Build history of the part. All positions in model axes, mm. A direction names the side the tool comes from. Round coordinates to 2 decimals unless told otherwise and drop trailing zeros. Order: outer loops, then holes, each group sorted by start corner. A loop starts at its lowest first (then second) coordinate and runs counter-clockwise, first axis right, second up. Notation, with made-up numbers: (35, -11.5) -> (67, -11.5) arc R17 cw to (67, 3.5) -> close; hole circle Ø10 at (2, 88.5). An arc over 180 degrees is marked (long way). Answer as a JSON object with one key per item and string values.
from build123d import *

# Parameters (mm, degrees)
EXTRUDE_1_DEPTH         = 3
SKETCH_2_R              = 1.35
CUT_EXTRUDE_1_DEPTH     = 2.444444444
SKETCH_3_R              = 1.35
CUT_EXTRUDE_2_DEPTH     = 0.555555556
HOLE_WIZARD_2_7_2_7_1_D = 2.7
SKETCH_6_R              = 1.65
CUT_EXTRUDE_3_DEPTH     = 64.035907885
CUT_EXTRUDE_4_DEPTH     = 1


with BuildPart() as part:
    # 草图1 → 凸台-拉伸1 (new body)
    with BuildSketch(Plane.XY.offset(3)):
        with BuildLine():
            Line((23.778016459, 8.467622986), (-52.596358319, 8.467622986))
            ThreePointArc((-52.596358319, 8.467622986), (-62.214907854, 3.590303351), (-52.451603626, -0.990377005))
            Line((-52.451603626, -0.990377005), (23.856567017, 0.468594516))
            ThreePointArc((23.856567017, 0.468594516), (27.777721585, 4.50700022), (23.778016459, 8.467622986))
        make_face()
    extrude(amount=-EXTRUDE_1_DEPTH)

    # 草图2 → 切除-拉伸1 (cut)
    with BuildSketch(Plane.XY.offset(3)):
        with Locations(Location((23.77801746, 4.467622995, 0), (0, 0, 180))):
            Circle(SKETCH_2_R)
    extrude(amount=-CUT_EXTRUDE_1_DEPTH, mode=Mode.SUBTRACT)

    # 草图3 → 切除-拉伸2 (cut)
    with BuildSketch(Plane(origin=(0, 0, 0), x_dir=(-1, 0, 0), z_dir=(0, 0, -1))):
        with Locations(Location((-23.778017455, 4.467823177, 0), (0, 0, 359.991504025))):
            Circle(SKETCH_3_R)
    extrude(amount=-CUT_EXTRUDE_2_DEPTH, mode=Mode.SUBTRACT)

    # Ø2.7 (2.7) 直径孔1 (through all)
    with Locations(Plane.XY.offset(3)):
        with Locations((-56.215609969, 3.682122995)):
            Hole(HOLE_WIZARD_2_7_2_7_1_D / 2)

    # 草图6 → 切除-拉伸3 (cut, through all)
    with BuildSketch(Plane.XY.offset(3)):
        with Locations((-56.215609969, 3.682122995)):
            Circle(SKETCH_6_R)
        with Locations((23.778017455, 4.467823177)):
            Circle(SKETCH_6_R)
    extrude(amount=-CUT_EXTRUDE_3_DEPTH, mode=Mode.SUBTRACT)

    # 草图7 → 切除-拉伸4 (cut)
    with BuildSketch(Plane.XY.offset(3)):
        with BuildLine():
            Line((-28.902991884, 4.643891928), (-29.217094448, 4.643891928))
            add(Edge.make_bspline(
                [(-29.217094448, 4.643891928), (-29.208584898, 4.679124412), (-29.191949422, 4.748001036), (-29.157251849, 4.846408297), (-29.119452594, 4.939531818), (-29.074063489, 5.025627892), (-29.024554735, 5.106426795), (-28.967832013, 5.180095919), (-28.906512291, 5.248508885), (-28.838687341, 5.309222122), (-28.76755868, 5.364199852), (-28.69212406, 5.411074909), (-28.613901166, 5.451399062), (-28.532348033, 5.484619294), (-28.447221862, 5.509644817), (-28.359292238, 5.527801623), (-28.268328738, 5.539592737), (-28.206581148, 5.5407435), (-28.175227461, 5.541327825)],
                knots=[0, 0, 0, 0, 1.162005537, 2.271625781, 3.343758855, 4.383309926, 5.390229558, 6.379919256, 7.361854164, 8.333198761, 9.295911338, 10.242430842, 11.177959212, 12.116337295, 13.062827104, 14.020064771, 14.994644689, 16, 16, 16, 16], degree=3))
            add(Edge.make_bspline(
                [(-28.175227461, 5.541327825), (-28.129544719, 5.539948595), (-28.039175708, 5.53722022), (-27.906412661, 5.512305783), (-27.778385842, 5.472880651), (-27.656496594, 5.418406924), (-27.543278162, 5.35121961), (-27.442541975, 5.271254874), (-27.355653464, 5.180055572), (-27.282759087, 5.079323008), (-27.225684088, 4.971667498), (-27.183597714, 4.860867341), (-27.157976033, 4.74718537), (-27.154655476, 4.670428091), (-27.152991884, 4.631972857)],
                knots=[0, 0, 0, 0, 1.083050992, 2.142477498, 3.193116406, 4.255571735, 5.30263384, 6.308962982, 7.297363603, 8.282367274, 9.249857812, 10.179914175, 11.08814088, 12, 12, 12, 12], degree=3))
            add(Edge.make_bspline(
                [(-27.152991884, 4.631972857), (-27.154155475, 4.594966063), (-27.156432443, 4.522549508), (-27.175766148, 4.416828011), (-27.208302411, 4.317186411), (-27.253372174, 4.223205249), (-27.311713724, 4.135480409), (-27.382386421, 4.053814518), (-27.465889082, 3.97784536), (-27.52916802, 3.934325887), (-27.561745891, 3.911920774)],
                knots=[0, 0, 0, 0, 1.024540389, 2.004866551, 2.965041327, 3.920577974, 4.882998113, 5.874504559, 6.905732034, 8, 8, 8, 8], degree=3))
            add(Edge.make_bspline(
                [(-27.561745891, 3.911920774), (-27.524514136, 3.893942602), (-27.450747262, 3.858322645), (-27.350196732, 3.788466887), (-27.258918857, 3.70781054), (-27.208015138, 3.644867887), (-27.182439, 3.613242889)],
                knots=[0, 0, 0, 0, 1.015518401, 2.012035669, 3.001164323, 4, 4, 4, 4], degree=3))
            add(Edge.make_bspline(
                [(-27.182439, 3.613242889), (-27.165597657, 3.590185138), (-27.132190761, 3.544447221), (-27.090955228, 3.470910795), (-27.053546113, 3.396559306), (-27.024395894, 3.3193999), (-27.001822027, 3.240326886), (-26.985685995, 3.15920449), (-26.975661854, 3.075966468), (-26.974226302, 3.019653988), (-26.973504705, 2.991347857)],
                knots=[0, 0, 0, 0, 1.025084078, 2.033381695, 3.024893161, 4.013698104, 4.991890475, 5.976764909, 6.982997093, 8, 8, 8, 8], degree=3))
            add(Edge.make_bspline(
                [(-26.973504705, 2.991347857), (-26.975299218, 2.942338136), (-26.9788798, 2.844549334), (-27.010883875, 2.700074613), (-27.060497115, 2.55884911), (-27.130954051, 2.423774271), (-27.21682156, 2.29739389), (-27.318978884, 2.184317581), (-27.436265293, 2.087118977), (-27.567070942, 2.005908749), (-27.70878807, 1.940990827), (-27.860363662, 1.895933384), (-28.019613716, 1.866587384), (-28.128821014, 1.863440515), (-28.184342045, 1.861840646)],
                knots=[0, 0, 0, 0, 0.955779014, 1.907060117, 2.875433937, 3.871313158, 4.872415639, 5.851225146, 6.836215519, 7.83643374, 8.849228613, 9.86973379, 10.916971861, 12, 12, 12, 12], degree=3))
            add(Edge.make_bspline(
                [(-28.184342045, 1.861840646), (-28.221761345, 1.862708859), (-28.29539005, 1.864417213), (-28.403633548, 1.876095814), (-28.506955248, 1.89742582), (-28.605494846, 1.926129125), (-28.699339882, 1.962520867), (-28.788203987, 2.007839565), (-28.872633881, 2.061151067), (-28.951832832, 2.123084655), (-29.0257914, 2.192365995), (-29.092544124, 2.270225005), (-29.153203917, 2.355222409), (-29.206146555, 2.448345465), (-29.253783508, 2.548390722), (-29.292964465, 2.656639221), (-29.327450033, 2.772123243), (-29.343483498, 2.852600983), (-29.351709833, 2.893891928)],
                knots=[0, 0, 0, 0, 1.048658725, 2.063410685, 3.046034179, 4.001477787, 4.936774919, 5.862367409, 6.792675028, 7.730719943, 8.675894397, 9.627829632, 10.600096036, 11.597688215, 12.626045268, 13.701542398, 14.82072376, 16, 16, 16, 16], degree=3))
            Line((-29.351709833, 2.893891928), (-29.037607269, 2.893891928))
            add(Edge.make_bspline(
                [(-29.037607269, 2.893891928), (-29.029423978, 2.866942915), (-29.013506765, 2.814524743), (-28.986412467, 2.739084437), (-28.955544195, 2.669926384), (-28.922429636, 2.606543262), (-28.88765119, 2.54831086), (-28.848736265, 2.496768991), (-28.80856712, 2.449653788), (-28.778287766, 2.423109176), (-28.763468647, 2.410117889)],
                knots=[0, 0, 0, 0, 1.198163088, 2.33053128, 3.407730985, 4.417276592, 5.372219308, 6.28897303, 7.162600585, 8, 8, 8, 8], degree=3))
            add(Edge.make_bspline(
                [(-28.763468647, 2.410117889), (-28.743872071, 2.395009556), (-28.704739408, 2.364839524), (-28.640971177, 2.326337895), (-28.573906291, 2.29297687), (-28.502091616, 2.267493174), (-28.427076846, 2.245915513), (-28.347649481, 2.231794994), (-28.264510264, 2.222106823), (-28.2077425, 2.221251891), (-28.17873307, 2.220815005)],
                knots=[0, 0, 0, 0, 0.946170439, 1.889420265, 2.845303464, 3.807233317, 4.801018734, 5.828864929, 6.890507805, 8, 8, 8, 8], degree=3))
            add(Edge.make_bspline(
                [(-28.17873307, 2.220815005), (-28.145979568, 2.22143091), (-28.081932921, 2.22263526), (-27.988478061, 2.233710966), (-27.899570614, 2.24984138), (-27.816197688, 2.274754363), (-27.737267181, 2.305535214), (-27.663885531, 2.34418362), (-27.595089425, 2.389528341), (-27.531760019, 2.4410675), (-27.474814512, 2.497488995), (-27.424674999, 2.556502066), (-27.382050337, 2.617857896), (-27.347666759, 2.681896016), (-27.320516209, 2.748351245), (-27.302033008, 2.817410075), (-27.289181493, 2.888507341), (-27.288134881, 2.93683631), (-27.287607269, 2.96119962)],
                knots=[0, 0, 0, 0, 1.217147791, 2.380027433, 3.494444702, 4.572153297, 5.609568379, 6.639424714, 7.649109417, 8.668170816, 9.669597737, 10.625200337, 11.543417969, 12.441394052, 13.322311151, 14.205496177, 15.095365482, 16, 16, 16, 16], degree=3))
            add(Edge.make_bspline(
                [(-27.287607269, 2.96119962), (-27.289137571, 2.993810959), (-27.292190559, 3.058871367), (-27.315499138, 3.154588942), (-27.353838003, 3.246812354), (-27.407510514, 3.333968144), (-27.472846243, 3.414744046), (-27.549211149, 3.486815528), (-27.637239378, 3.546285619), (-27.718259247, 3.587374276), (-27.790024403, 3.615411351), (-27.851439788, 3.634086315), (-27.920196391, 3.649899971), (-27.99546274, 3.664612242), (-28.077805957, 3.677133591), (-28.167136394, 3.687575406), (-28.263472156, 3.695930447), (-28.330163322, 3.699661543), (-28.364530346, 3.701584236)],
                knots=[0, 0, 0, 0, 1.07054697, 2.135767047, 3.216561865, 4.33974944, 5.486079747, 6.621378074, 7.775625952, 8.963672916, 9.598146892, 10.304877434, 11.070270905, 11.915000392, 12.823868403, 13.805723172, 14.86925407, 16, 16, 16, 16], degree=3))
            Line((-28.364530346, 3.701584236), (-28.364530346, 4.060558595))
            add(Edge.make_bspline(
                [(-28.364530346, 4.060558595), (-28.32122918, 4.061293398), (-28.236412834, 4.062732698), (-28.112518529, 4.080140709), (-27.994045217, 4.104221337), (-27.883618475, 4.141106529), (-27.782969761, 4.183946826), (-27.695650159, 4.233799035), (-27.622883012, 4.289213785), (-27.565021941, 4.351046394), (-27.521492712, 4.417361441), (-27.489665914, 4.486478099), (-27.470865588, 4.55900216), (-27.468355921, 4.608496828), (-27.467094448, 4.633375101)],
                knots=[0, 0, 0, 0, 1.321986639, 2.589447074, 3.816329219, 5.01088745, 6.139805852, 7.153945165, 8.075214402, 8.924034688, 9.728124013, 10.488707548, 11.240355623, 12, 12, 12, 12], degree=3))
            add(Edge.make_bspline(
                [(-27.467094448, 4.633375101), (-27.467508859, 4.651652846), (-27.46833331, 4.688015553), (-27.478730588, 4.741140622), (-27.494354629, 4.792641568), (-27.515834358, 4.842299378), (-27.544584557, 4.889769652), (-27.578990544, 4.935457101), (-27.619958644, 4.97910088), (-27.666904091, 5.019781199), (-27.717315896, 5.058550437), (-27.772565671, 5.091464074), (-27.830987546, 5.119609136), (-27.892646201, 5.142818638), (-27.957741731, 5.160277926), (-28.025968289, 5.172813767), (-28.097455972, 5.180651422), (-28.146227704, 5.181779838), (-28.171020731, 5.182353466)],
                knots=[0, 0, 0, 0, 0.884392785, 1.759457502, 2.611959086, 3.489218968, 4.37281399, 5.2945488, 6.255912374, 7.266815255, 8.301784654, 9.332968512, 10.37626691, 11.440494194, 12.520033166, 13.637162961, 14.798855837, 16, 16, 16, 16], degree=3))
            add(Edge.make_bspline(
                [(-28.171020731, 5.182353466), (-28.210872399, 5.180962104), (-28.288711975, 5.178244451), (-28.400926892, 5.154441437), (-28.505246226, 5.116463354), (-28.584984892, 5.071130334), (-28.643867467, 5.026379901), (-28.685944405, 4.987297514), (-28.727264915, 4.94386469), (-28.765110592, 4.893406315), (-28.803384569, 4.839339525), (-28.83822913, 4.778915843), (-28.872088822, 4.713711449), (-28.892491372, 4.667615815), (-28.902991884, 4.643891928)],
                knots=[0, 0, 0, 0, 1.472543308, 2.876219568, 4.221790263, 5.565193594, 6.249813518, 6.953379497, 7.687249741, 8.463570142, 9.283606569, 10.136032583, 11.040678096, 12, 12, 12, 12], degree=3))
        make_face()
    extrude(amount=-CUT_EXTRUDE_4_DEPTH, mode=Mode.SUBTRACT)


solid = part.part
1) Cut at B-B, the plane x = -43.5. Give the cut face in (y, z).
Checked values:
{"outline": "(-0.82, 0) -> (8.47, 0) -> (8.47, 3) -> (-0.82, 3) -> close"}
2) Cut at C-C, the plane x = 6.5. Give the cut face in (y, z).
Checked values:
{"outline": "(0.14, 0) -> (8.47, 0) -> (8.47, 3) -> (0.14, 3) -> close"}
3) Probe L1, parallel to X at y = 4.25, z = 1.55; L2, parallel to X at y = 3.25, z = 0.3; L3, parallel to X at y = 4.75, z = 2.2. List the from-to ranges inside material, lowest first. Write a range as from..to.
Checked values:
{"L1": "x = -62.19..-57.76, -54.67..22.14, 25.41..27.77", "L2": "x = -62.2..-57.81, -54.62..22.66, 24.89..27.59", "L3": "x = -62.12..-57.47, -54.96..-29.19, -28.85..-27.48, -27.16..22.15, 25.4..27.77"}
4) Which spindle directions (+Z, -Z, +X, -X, +Y, -Y) get a long thin tool onto all of the face, cutting with end or side? Do faces 1 (the face through (-57.864, 3.755, 1.521)), 2 (the face through (-14, 8.468, 2)). Say none if no direction does.
Checked values:
{"face 1": "+Z, -Z", "face 2": "+Z, -Z, +X, +Y"}
5) Pull direction Y, two halves, no side cores. Call faces 3 (the face through (-28.07, 3.85, 2)), 4 (the face through (-18, 4, 0)), 5 (the face through (27.778, 4.42, 1.521)): pulls with the +Y half, pulls with the -Y half, needs draft (parallel to the pull), parting line crosses it, or undercut.
Checked values:
{"face 3": "undercut", "face 4": "needs draft", "face 5": "parting line crosses it"}
6) Flat gauge pins, fed straight in: pin 1 Ø4 at (x, y) = (-56.22, 3.68) entering from +Z; pin 2 Ø1 at (x, z) = (-14, 2) entering from -Y; pin 3 Ø1 at (x, z) = (1.5, 1.5) entering from +Y; pin 4 Ø1.5 at (y, z) = (7.5, 0.5) entering from -X. Where does each tip first touch, or does it go through?
Checked values:
{"pin 1": "stops at z = 3", "pin 2": "stops at y = -0.26", "pin 3": "stops at y = 8.47", "pin 4": "stops at x = -61.37"}
7) Cut at A-A, the plane z = 1.3. Give the cut face in (x, y).
Checked values:
{"outline": "(-52.6, 8.47) arc R6 ccw (long way) to (-52.45, -0.99) -> (23.86, 0.47) arc R4 ccw to (23.78, 8.47) -> close; hole circle Ø3.3 at (-56.22, 3.68); hole circle Ø3.3 at (23.78, 4.47)"}
